from build123d import *

# Parameters (mm, degrees)
SKETCH1_W           = 76.2
SKETCH1_H           = 76.2
SKETCH1_R           = 2.54
BOSS_EXTRUDE1_DEPTH = 6.35


with BuildPart() as part:
    # Sketch1 → Boss-Extrude1 (new body)
    with BuildSketch(Plane(origin=(0, 0, 0), x_dir=(1, 0, 0), z_dir=(0, 1, 0))):
        Rectangle(SKETCH1_W, SKETCH1_H)
        with BuildLine():
            Line((2.609105575, -0.625751054), (0.975970434, -2.4992955))
            ThreePointArc((0.975970434, -2.4992955), (-2.022556476, 1.763026259), (2.609105575, -0.625751054))
        make_face(mode=Mode.SUBTRACT)
        with Locations(Location((-29.120418144, -29.120418144, 0), (0, 0, 270))):
            Circle(SKETCH1_R, mode=Mode.SUBTRACT)
        with Locations(Location((29.120418144, 29.120418144, 0), (0, 0, 270))):
            Circle(SKETCH1_R, mode=Mode.SUBTRACT)
        with Locations(Location((29.120418144, -29.120418144, 0), (0, 0, 270))):
            Circle(SKETCH1_R, mode=Mode.SUBTRACT)
        with Locations(Location((-29.120418144, 29.120418144, 0), (0, 0, 270))):
            Circle(SKETCH1_R, mode=Mode.SUBTRACT)
    extrude(amount=BOSS_EXTRUDE1_DEPTH)


solid = part.part
Read the model definition and answer for the solid it produces. Units are mm, in the model's axes. A direction names the side the tool comes from. Round coordinates to 2 decimals unless told otherwise and drop trailing zeros. Loops run counter-clockwise (first coordinate to the right, second up) from the corner with the lowest first, then second, coordinate; pieces in that order, holes last. Notation, with made-up numbers: (18, 57.25) - (76, 57.25) arc R11 cw to (76, 70.25) - close; hole circle Ø5 at (68.5, -13). An arc over 180 degrees is marked (long way). One line per question, with ' | ' between items. Start each with the question number.
Q1. Section B-B on y = 3.5 is taken. Give the vertices of the cut face in (x, z), plus the area to 3 significant figures.
Q2. For faces 4 (the flat face through (38.1, 3, 1)), 5 (the flat face through (1.804, 3.131, 1.549)), determine the directions among +Z, -Z, +X, -X, +Y, -Y from which every point of the face is accessible in a straight line to the end or side of a thin tool.
Q3. Find the intervals of material crossed by L1, parallel to X at y = 1.5, z = 0; L2, parallel to X at y = 2.5, z = 27, in increasing order.
Q4. Section A-A on x = 0 is taken. Give the vertices of the cut face in (y, z), plus the area to 3 significant figures.
Q5. Section C-C on z = 27.5 is taken. Give the vertices of the cut face in (x, y), plus the area to 3 significant figures.
Q6. For a pull along Z with two mould halves and no side action, classify faces 1 (the flat face through (-1, 3, 38.1)), 2 (the flat face through (8, 0, -1)), 3 (the cylindrical face through (-30.666, 3.131, 27.105)) as +Z half, -Z half, draft (parallel to the pull), parting line (faces both ways), or undercut.
Q7. A flat-ended cylindrical pin translates along its axis: pin 1 (6.5 mm diameter, centred on x = -29.12, z = -29.12, fed in from +Y). Find the tip coordinate at first contact, or state that the pin passes through.
Q8. Section D-D on x = 27.5 is taken. Give the vertices of the cut face in (y, z).
Established:
1) outline: (-38.1, -38.1) - (38.1, -38.1) - (38.1, 38.1) - (-38.1, 38.1) - close; hole circle Ø5.08 at (-29.12, -29.12); hole circle Ø5.08 at (-29.12, 29.12); hole (0.98, 2.5) arc R2.68 ccw (long way) to (2.61, 0.63) - close; hole circle Ø5.08 at (29.12, -29.12); hole circle Ø5.08 at (29.12, 29.12) | area: 5,700 mm²
2) face 4: +Z, -Z, +X, +Y, -Y | face 5: +Y, -Y
3) L1: -38.1 to -2.68, 2.68 to 38.1 | L2: -38.1 to -30.52, -27.72 to 27.72, 30.52 to 38.1
4) outline: (0, -38.1) - (6.35, -38.1) - (6.35, -2.68) - (0, -2.68) - close; (0, 2.68) - (6.35, 2.68) - (6.35, 38.1) - (0, 38.1) - close | area: 450 mm²
5) outline: (-38.1, 0) - (-31.08, 0) - (-31.08, 6.35) - (-38.1, 6.35) - close; (-27.16, 0) - (27.16, 0) - (27.16, 6.35) - (-27.16, 6.35) - close; (31.08, 0) - (38.1, 0) - (38.1, 6.35) - (31.08, 6.35) - close | area: 434 mm²
6) face 1: +Z half | face 2: draft | face 3: undercut
7) pin 1: y = 6.35
8) outline: (0, -38.1) - (6.35, -38.1) - (6.35, -31.08) - (0, -31.08) - close; (0, -27.16) - (6.35, -27.16) - (6.35, 27.16) - (0, 27.16) - close; (0, 31.08) - (6.35, 31.08) - (6.35, 38.1) - (0, 38.1) - close
